Geometry: see drawing. Coordinates: mm, zero at the bounding-box minimum. A direction names the side the tool comes from. Round coordinates to 2 decimals unless told otherwise and drop trailing zeros. Order: outer loops, then holes, each group sorted by start corner. A loop starts at its lowest first (then second) coordinate and runs counter-clockwise, first axis right, second up. Notation, with made-up numbers: (-10, 4) -> (33, 4) arc R20 cw to (33, 14) -> close; hole circle Ø2 at (30, 12). An arc over 180 degrees is marked (long way). Answer as CSV lines item,"result". Start each with the question number.
(1) Section query A-A (z = 105). Output: boundary loops of the cut face in (x, y) (1 decimal).
(2) Section query D-D (z = 418). Output: boundary loops of the cut face in (x, y).
(3) Line query: line 1 along Y through (x, z) = (185.5, 308); line 2 along X through (y, z) = (157, 140.5) (1 decimal); line 3 along Z through (x, y) = (812, 373.5). Output: solid intervals per line, ascending. Write a range as from..to.
(4) Section query C-C (y = 441). Output: boundary loops of the cut face in (x, z) (1 decimal), plus the area to 3 significant figures.
(5) Section query B-B (x = 825). Output: boundary loops of the cut face in (y, z).
(6) Set-up query: the marked faces 4, 5 and 6. Return all of +Z, -Z, +X, -X, +Y, -Y with unobstructed straight access to the full face (end or side cutting, diameter ignored); none if empty.
(7) Contact query for a flat-ended pin moving along its axis: P1, Ø3, axis at x = 381, y = 692.5, coming from the +Z side. Output: stop coordinate, or through.
(8) Pull-direction query (Y, two-part tool) for the marked faces 1, 2 and 3; classes: +Y half, -Y half, draft (parallel to the pull), parting line (faces both ways), or undercut.
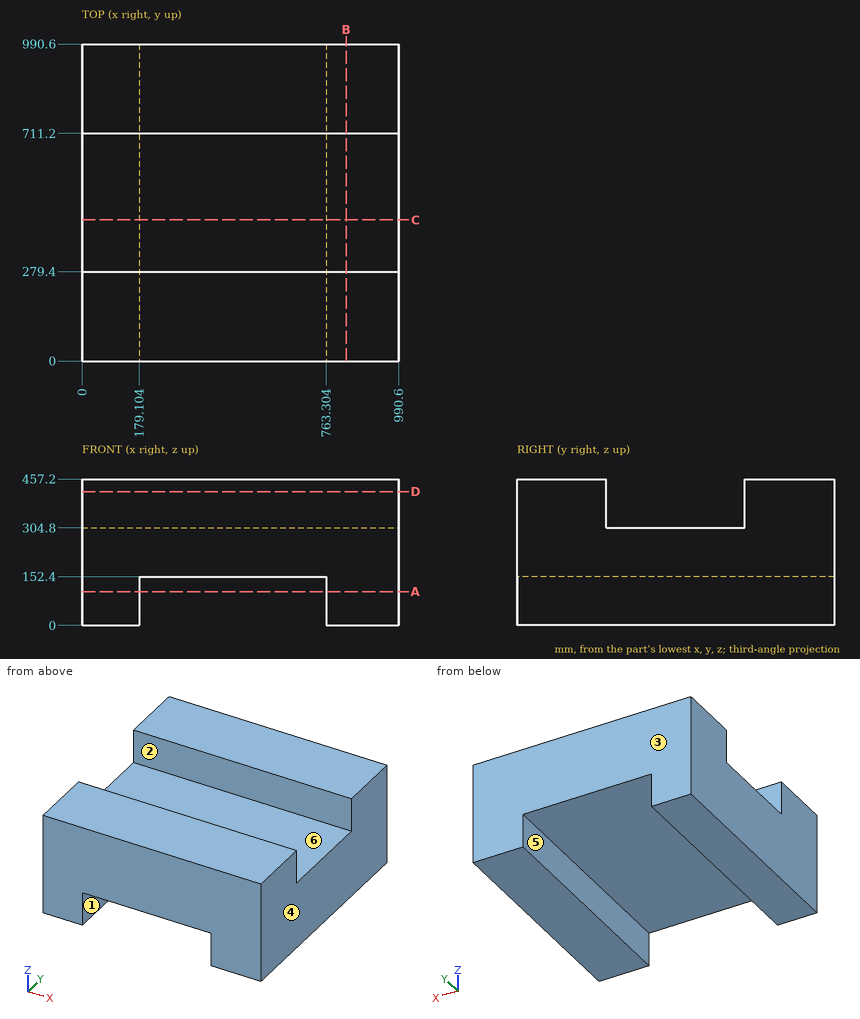
Answer block:
1,outline,"(0, 0) -> (179.1, 0) -> (179.1, 990.6) -> (0, 990.6) -> close; (763.3, 0) -> (990.6, 0) -> (990.6, 990.6) -> (763.3, 990.6) -> close"
2,outline,"(0, 0) -> (990.6, 0) -> (990.6, 279.4) -> (0, 279.4) -> close; (0, 711.2) -> (990.6, 711.2) -> (990.6, 990.6) -> (0, 990.6) -> close"
3,line 1,"0..279.4, 711.2..990.6"
3,line 2,"0..179.1, 763.3..990.6"
3,line 3,"0..304.8"
4,outline,"(0, 0) -> (179.1, 0) -> (179.1, 152.4) -> (763.3, 152.4) -> (763.3, 0) -> (990.6, 0) -> (990.6, 304.8) -> (0, 304.8) -> close"
4,area,"213,000 mm2"
5,outline,"(0, 0) -> (990.6, 0) -> (990.6, 457.2) -> (711.2, 457.2) -> (711.2, 304.8) -> (279.4, 304.8) -> (279.4, 457.2) -> (0, 457.2) -> close"
6,face 4,"+Z, -Z, +X, +Y, -Y"
6,face 5,"-Z, +Y, -Y"
6,face 6,"+Z, +X, -X"
7,P1,"z = 304.8"
8,face 1,"draft"
8,face 2,"undercut"
8,face 3,"+Y half"
